Geometry check sheet. Reference: drawing and pictorial views, mm from the part's lowest x, y, z. A direction names the side the tool comes from. Coordinates: 2 decimals unless noted, no trailing zeros. Return JSON: item names as keys, results as strings.
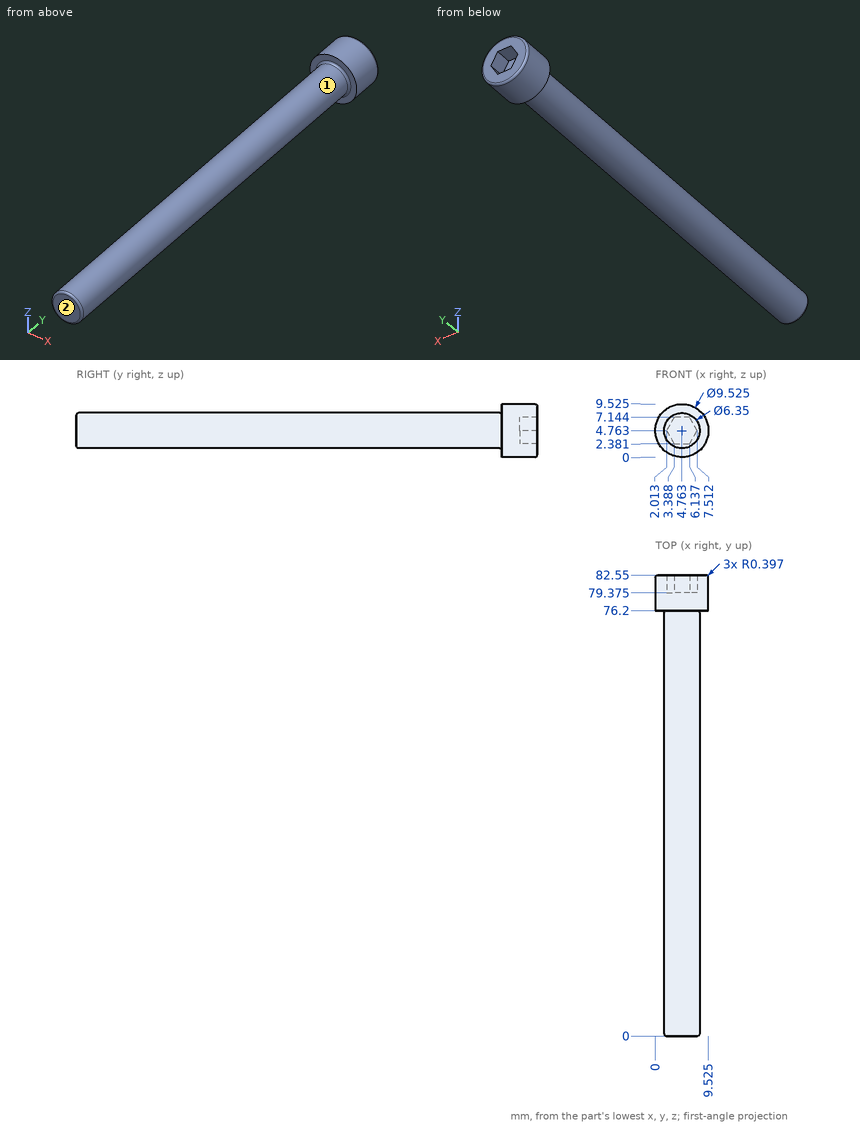
Q1. Tool access check on the marked faces 1 and 2. Record the directions out of +Z, -Z, +X, -X, +Y, -Y that give a thin tool (end or side, any length) a straight path to the whole face; none if there is none.
Values:
{"face 1": "-Y", "face 2": "+Z, -Z, +X, -X, -Y"}
Q2. Go/stop test with flat-tipped pins: pin 1 (1.5 mm diameter, centred on x = 4, z = 3, fed in from +Y); pin 2 (1 mm diameter, centred on x = 6, y = 69, fed in from -Z) (1 decimal); pin 3 (4 mm diameter, centred on y = 46.5, z = 2.5, fed in from +X); pin 4 (3 mm diameter, centred on x = 4, y = 60.5, fed in from -Z). Record where each tip stops, or that it passes through.
Values:
{"pin 1": "y = 82.55", "pin 2": "z = 1.7", "pin 3": "x = 7.93", "pin 4": "z = 1.59"}
Q3. Material ranges on line 1 along Y through (x, z) = (4.25, 3) (1 decimal); line 2 along Y through (x, z) = (4, 8.5); line 3 along X through (y, z) = (48.5, 3.25) (1 decimal), recorded low to high.
Values:
{"line 1": "0 to 79.4", "line 2": "76.2 to 82.55", "line 3": "2 to 7.6"}
